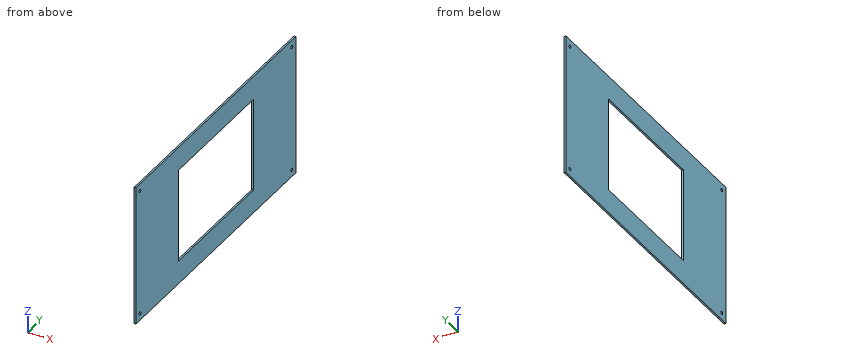
from build123d import *

# Parameters (mm, degrees)
SKETCH1_W           = 500
SKETCH1_H           = 250
SKETCH1_R           = 2.8
BOSS_EXTRUDE1_DEPTH = 3.175
SKETCH2_W           = 235.5
SKETCH2_H           = 166.5
CUT_EXTRUDE1_DEPTH  = 280.526529376


with BuildPart() as part:
    # Sketch1 → Boss-Extrude1 (new body)
    with BuildSketch(Plane.YZ):
        Rectangle(SKETCH1_W, SKETCH1_H)
        with Locations(Location((-237.5, 112.5, 0), (0, 0, 270))):
            Circle(SKETCH1_R, mode=Mode.SUBTRACT)
        with Locations(Location((237.5, 112.5, 0), (0, 0, 90))):
            Circle(SKETCH1_R, mode=Mode.SUBTRACT)
        with Locations(Location((237.5, -112.5, 0), (0, 0, 270))):
            Circle(SKETCH1_R, mode=Mode.SUBTRACT)
        with Locations(Location((-237.5, -112.5, 0), (0, 0, 90))):
            Circle(SKETCH1_R, mode=Mode.SUBTRACT)
    extrude(amount=BOSS_EXTRUDE1_DEPTH)

    # Sketch2 → Cut-Extrude1 (cut, through all)
    with BuildSketch(Plane.YZ.offset(3.175)):
        Rectangle(SKETCH2_W, SKETCH2_H)
    extrude(amount=-CUT_EXTRUDE1_DEPTH, mode=Mode.SUBTRACT)


solid = part.part
Source: CAD feature listing. Evaluate the final solid. Frame: model axes, mm. Give positions to 0.01 mm unless a question says otherwise; leave off trailing zeros. Write each loop counter-clockwise with the first axis right and the second up, starting at its lowest first coordinate (ties: lowest second). Pieces come first, ordered by that corner, then holes. Notation, with made-up numbers: (2, 3) - (39, 3) arc R17 cw to (39, 36) - close; hole circle Ø4 at (44.25, -2.75). An arc over 180 degrees is marked (long way). Write item = value, one per line. Start each with the question number.
Q1. Pin query (flat end, axial travel): pin 1 Ø4 at (y, z) = (-117.5, 51) entering from +X (3 decimals). Return the tip coordinate at first contact, or that it passes through.
Q2. Cut plane C-C, the plane x = 2.6. Return loops of the section in (y, z).
Q3. Cut plane A-A, the plane y = -13. Return loops of the section in (x, z) (3 decimals), then the cut area to 3 significant figures.
Q4. Cut plane B-B, the plane z = -46. Return loops of the section in (x, y) (3 decimals), then the cut area to 3 significant figures.
Q5. Material intervals for probe 1 along Y at (x, z) = (2.15, -112.5); probe 2 along Z at (x, y) = (0.95, -237.5); probe 3 along Y at (x, z) = (2.5, 32.5), sorted ascending.
Computed values:
q1.pin_1 = 3.175
q2.outline = (-250, -125) - (250, -125) - (250, 125) - (-250, 125) - close; hole circle Ø5.6 at (-237.5, -112.5); hole circle Ø5.6 at (-237.5, 112.5); hole (-117.75, -83.25) - (117.75, -83.25) - (117.75, 83.25) - (-117.75, 83.25) - close; hole circle Ø5.6 at (237.5, -112.5); hole circle Ø5.6 at (237.5, 112.5)
q3.outline = (0, -125) - (3.175, -125) - (3.175, -83.25) - (0, -83.25) - close; (0, 83.25) - (3.175, 83.25) - (3.175, 125) - (0, 125) - close
q3.area = 265 mm²
q4.outline = (0, -250) - (3.175, -250) - (3.175, -117.75) - (0, -117.75) - close; (0, 117.75) - (3.175, 117.75) - (3.175, 250) - (0, 250) - close
q4.area = 840 mm²
q5.probe_1 = -250 to -240.3, -234.7 to 234.7, 240.3 to 250
q5.probe_2 = -125 to -115.3, -109.7 to 109.7, 115.3 to 125
q5.probe_3 = -250 to -117.75, 117.75 to 250
